Autodesk Inventor part; units mm, degrees
ref_plane "YZ Plane" through (0, 0, 0) normal (1, 0, 0) x (0, 1, 0)
ref_plane "XZ Plane" through (0, 0, 0) normal (0, 1, 0) x (-1, 0, 0)
ref_plane "XY Plane" through (0, 0, 0) normal (0, 0, 1) x (1, 0, 0)
sketch "Skizze1" plane through (0, 0, 0) normal (0, 1, 0) x (-1, 0, 0)
  line L0 (-19.75, -14.75) -> (19.75, -14.75)
  line L1 (19.75, -14.75) -> (19.75, 14.75)
  line L2 (19.75, 14.75) -> (-19.75, 14.75)
  line L3 (-19.75, 14.75) -> (-19.75, -14.75)
  line L4 (0, -20.65) -> (0, 20.65)
  line L5 (27.65, 0) -> (-27.65, 0)
  point P0 (0, 0)
  dimension "d0" = 39.5
  dimension "d1" = 29.5
extrude "Extrusion1" add sketch "Skizze1" along normal blind 6
sketch "Skizze2" plane through (0, 6, 0) normal (0, 1, 0) x (1, 0, 0)
  line L0 (19.75, 14.75) -> (-19.75, 14.75)
  line L1 (-19.75, 14.75) -> (-11.75, 14.75)
  line L2 (-12, 12.75) -> (-12, 7)
  line L3 (-12, 7) -> (-17.75, 7)
  line L4 (-19.75, 6.75) -> (-19.75, 14.75)
  line L5 (19.75, 14.75) -> (10.75, 14.75)
  line L6 (12, 12.75) -> (12, 7)
  line L7 (12, 7) -> (17.75, 7)
  line L8 (19.75, 10.8731) -> (19.75, 14.75)
  line L9 (-19.75, -14.75) -> (19.75, -14.75)
  line L10 (-19.75, -14.75) -> (-11.75, -14.75)
  line L11 (-12, -12.75) -> (-12, -7)
  line L12 (-12, -7) -> (-17.75, -7)
  line L13 (-19.75, -6.75) -> (-19.75, -14.75)
  line L14 (19.75, -14.75) -> (11.75, -14.75)
  line L15 (12, -12.75) -> (12, -7)
  line L16 (12, -7) -> (17.75, -7)
  line L17 (19.75, -6.75) -> (19.75, -14.75)
  circle A0 centre (-14.75, 9.75) radius 1.75
  circle A1 centre (-14.75, -9.75) radius 1.75
  circle A2 centre (14.75, -9.75) radius 1.75
  circle A3 centre (14.75, 9.75) radius 1.75
  line L18 (-19.75, 14.75) -> (-19.75, -14.75)
  line L19 (-19.75, 14.75) -> (19.75, 14.75)
  line L20 (19.75, 14.75) -> (19.75, -14.75)
  line L21 (19.75, -14.75) -> (-19.75, -14.75)
  line L22 (-19.75, -14.75) -> (-19.75, 14.75)
  line L23 (17.75, 12.75) -> (-17.75, 12.75)
  line L24 (-17.75, 12.75) -> (-17.75, -12.75)
  line L25 (-17.75, -12.75) -> (17.75, -12.75)
  line L26 (17.75, 12.75) -> (17.75, -12.75)
  point P0 (0, 0)
  dimension "d12" = 3.5
  dimension "d13" = 5
  dimension "d14" = 5
  dimension "d15" = 3.5
  dimension "d16" = 5
  dimension "d17" = 5
  dimension "d18" = 3.5
  dimension "d19" = 5
  dimension "d20" = 5
  dimension "d21" = 3.5
  dimension "d22" = 5
  dimension "d23" = 5
  dimension "d24" = 2
  dimension "d25" = 2
  dimension "d28" = 2
  dimension "d29" = 2
  dimension "d30" = 7.75
  dimension "d31" = 7.75
  dimension "d35" = 7.75
  dimension "d36" = 7.75
  dimension "d37" = 7.75
  dimension "d38" = 7.75
  dimension "d39" = 7.75
  dimension "d40" = 7.75
sketch "Skizze3" plane through (0, 6, 0) normal (0, 1, 0) x (1, 0, 0)
  circle A0 centre (5.25, 0) radius 7.7
  line L0 (19.75, -14.75) -> (19.75, 14.75)
  line L1 (19.75, 14.75) -> (-19.75, 14.75)
  point P0 (0, 0)
  dimension "d32" = 15.4
  dimension "d33" = 14.5
  dimension "d34" = 14.75
extrude "Extrusion2" add sketch "Skizze2" along normal blind 31.5 contours L8 L20 L17 L9 L13 L18 L4 L0
extrude "Extrusion3" cut sketch "Skizze3" against normal blind 4
sketch "Skizze4" plane through (5.25, 2, 0) normal (0, 1, 0) x (1, 0, 0)
  circle A0 centre (0, 0) radius 5.3
  point P0 (-5.25, 0)
  dimension "d45" = 10.6
extrude "Extrusion4" cut sketch "Skizze4" against normal up to surface (2 mm away)
extrude "Extrusion5" add sketch "Skizze2" along normal blind 31.5 contours L26 L25 L15 L16
extrude "Extrusion6" add sketch "Skizze2" along normal blind 31.5 contours L2 L3 L24 L23 | L23 L26 L7 L6 | L12 L11 L25 L24
extrude "Extrusion7" cut sketch "Skizze2" against normal up to surface (6 mm away) contours A0 | A1 | A2 | A3
fillet "Rundung1" radius 3.5 4 edges at (-12, 21.75, -7) (12, 21.75, -7) (-12, 21.75, 7) (12, 21.75, 7)
fillet "Rundung2" radius 4 4 edges at (19.75, 18.75, 14.75) (19.75, 18.75, -14.75) (-19.75, 18.75, -14.75) (-19.75, 18.75, 14.75)
sketch "Skizze5" plane through (-15.75, 0, 14.75) normal (0, 0, 1) x (1, 0, 0)
  line L0 (3.75, 34) -> (27.75, 34)
  line L1 (27.75, 34) -> (27.75, 17.5)
  line L2 (27.75, 17.5) -> (3.75, 17.5)
  line L3 (3.75, 17.5) -> (3.75, 34)
  line L4 (0, 37.5) -> (31.5, 37.5)
  line L5 (-4, 37.5) -> (-4, 0)
  line L6 (35.5, 0) -> (35.5, 37.5)
  point P0 (15.75, 0)
  dimension "d56" = 16.5
  dimension "d57" = 3.5
  dimension "d58" = 7.75
  dimension "d59" = 7.75
sketch "Skizze6" plane through (15.75, 0, -14.75) normal (0, 0, -1) x (-1, 0, 0)
  line L0 (31.25, 6) -> (27.75, 6)
  line L1 (3.75, 34) -> (27.75, 34)
  line L2 (27.75, 34) -> (27.75, 6)
  line L3 (27.75, 6) -> (3.75, 6)
  line L4 (3.75, 6) -> (3.75, 34)
  line L5 (0, 37.5) -> (31.5, 37.5)
  point P0 (15.75, 0)
  dimension "d60" = 3.5
extrude "Extrusion8" cut sketch "Skizze6" against normal up to surface (2 mm away)
extrude "Extrusion9" cut sketch "Skizze5" against normal up to surface (2 mm away)
sketch "Skizze7" plane through (-19.75, 0, -10.75) normal (-1, 0, 0) x (0, 0, 1)
  line L0 (3.25, 34) -> (17.25, 34)
  line L1 (17.25, 34) -> (17.25, 17.5)
  line L2 (17.25, 17.5) -> (3.25, 17.5)
  line L3 (3.25, 17.5) -> (3.25, 34)
  line L4 (-4, 37.5) -> (-4, 0)
  line L5 (0, 37.5) -> (21.5, 37.5)
  point P0 (10.75, 0)
  dimension "d65" = 14
  dimension "d66" = 16.5
  dimension "d67" = 7.25
  dimension "d68" = 3.5
extrude "Extrusion10" cut sketch "Skizze7" against normal up to surface (2 mm away)
sketch "Skizze8" plane through (19.75, 0, 10.75) normal (1, 0, 0) x (0, 0, -1)
  line L0 (3.25, 34) -> (17.25, 34)
  line L1 (17.25, 34) -> (17.25, 17.5)
  line L2 (17.25, 17.5) -> (3.25, 17.5)
  line L3 (3.25, 17.5) -> (3.25, 34)
  line L4 (-4, 37.5) -> (-4, 0)
  line L5 (0, 37.5) -> (21.5, 37.5)
  point P0 (10.75, 0)
  dimension "d71" = 14
  dimension "d72" = 16.5
  dimension "d73" = 7.25
  dimension "d74" = 3.5
extrude "Extrusion11" cut sketch "Skizze8" against normal up to surface (2 mm away)
sketch "Skizze12" plane through (15.75, 0, -14.75) normal (0, 0, -1) x (-1, 0, 0)
  line L0 (27.75, 34) -> (3.75, 34)
  line L1 (27.75, 6) -> (27.75, 37.5)
  line L2 (3.75, 34) -> (27.75, 34)
  line L3 (27.75, 34) -> (27.75, 37.5)
  line L4 (27.75, 37.5) -> (3.75, 37.5)
  line L5 (3.75, 37.5) -> (3.75, 34)
  point P0 (15.75, 0)
extrude "Extrusion14" cut sketch "Skizze12" against normal up to surface (2 mm away)
sketch "Skizze13" plane through (12, 37.5, 12.75) normal (0, 0, -1) x (-1, 0, 0)
  line L0 (0, 0) -> (0, -31.5)
  line L1 (24, -31.5) -> (24, 0)
  line L2 (0, -3.5027) -> (24, -3.5027)
  line L3 (24, -3.5027) -> (24, 0)
  line L4 (24, 0) -> (0, 0)
  line L5 (0, 0) -> (0, -3.5027)
  point P0 (12, -37.5)
  point P1 (24, -3.5027)
extrude "Extrusion15" cut sketch "Skizze13" against normal up to surface (2 mm away)
sketch "Skizze14" plane through (-15.75, 0, 14.75) normal (0, 0, 1) x (1, 0, 0)
  line L0 (3.75, 6) -> (3.75, 17.5)
  line L1 (27.75, 17.5) -> (27.75, 6)
  line L2 (3.75, 17.5) -> (27.75, 17.5)
  line L3 (27.75, 17.5) -> (27.75, 6)
  line L4 (27.75, 6) -> (3.75, 6)
  line L5 (3.75, 6) -> (3.75, 17.5)
  point P0 (15.75, 0)
  point P1 (27.75, 17.5)
extrude "Extrusion16" cut sketch "Skizze14" against normal up to surface (2 mm away)
sketch "Skizze15" plane through (-19.75, 0, -10.75) normal (-1, 0, 0) x (0, 0, 1)
  point P0 (10.75, 0)
sketch "Skizze16" plane through (-17.75, 6, 7) normal (1, 0, 0) x (0, 0, -1)
  line L0 (14, 0) -> (0, 0)
  line L1 (14, 11.5) -> (14, 28)
  line L2 (0, 0) -> (14, 0)
  line L3 (14, 0) -> (14, 11.5)
  line L4 (14, 11.5) -> (0, 11.5)
  line L5 (0, 11.5) -> (0, 0)
  line L6 (0, 31.5) -> (14, 31.5)
  line L7 (14, 28) -> (0, 28)
  line L8 (0, 28) -> (0, 31.5)
  line L9 (0, 31.5) -> (14, 31.5)
  line L10 (14, 31.5) -> (14, 28)
  point P0 (7, -6)
extrude "Extrusion17" cut sketch "Skizze16" against normal up to surface (2 mm away) contours L7 L8 L6 L10
extrude "Extrusion18" cut sketch "Skizze16" against normal up to surface (2 mm away) contours L0 L5 L4 L3
sketch "Skizze17" plane through (-17.75, 34, 6.5) normal (0, 0, -1) x (-1, 0, 0)
  line L0 (0, 0) -> (2, 0)
  line L1 (2, 0) -> (2, -16.5)
  line L2 (0, 0) -> (2, 0)
  line L3 (2, 0) -> (2, -16.5)
  line L4 (2, -16.5) -> (0, -16.5)
  line L5 (0, -16.5) -> (0, 0)
  point P0 (-17.75, -34)
extrude "Extrusion19" cut sketch "Skizze17" against normal blind 0.5
sketch "Skizze18" plane through (17.75, 6, -7) normal (-1, 0, 0) x (0, 0, 1)
  line L0 (14, 28) -> (14, 31.5)
  line L1 (0.5, 28) -> (14, 28)
  line L2 (14, 31.5) -> (0.5, 31.5)
  line L3 (0.5, 31.5) -> (0.5, 28)
  line L4 (0.5, 28) -> (14, 28)
  line L5 (14, 28) -> (14, 31.5)
  line L6 (14, 0) -> (0, 0)
  line L7 (14.5, 11.5) -> (14, 11.5)
  line L8 (0, 0) -> (14, 0)
  line L9 (14, 0) -> (14, 11.5)
  line L10 (14, 11.5) -> (0, 11.5)
  line L11 (0, 11.5) -> (0, 0)
  point P0 (7, -6)
extrude "Extrusion20" cut sketch "Skizze18" against normal up to surface (2 mm away) contours L6 L11 L10 L9
extrude "Extrusion21" cut sketch "Skizze18" against normal up to surface (2 mm away) contours L1 L3 L2 L0
sketch "Skizze19" plane through (17.75, 37.5, -6.5) normal (0, 0, 1) x (1, 0, 0)
  line L0 (0, -20) -> (0, 0)
  line L1 (2, 0) -> (2, -20)
  line L2 (0, -20) -> (2, -20)
  line L3 (2, -20) -> (2, 0)
  line L4 (2, 0) -> (0, 0)
  line L5 (0, 0) -> (0, -20)
  point P0 (-17.75, -37.5)
extrude "Extrusion22" cut sketch "Skizze19" against normal blind 0.5
properties part number "_3D-Druck"
Verification items for the finished model (mm, model axes). A direction names the side the tool comes from. Give positions to 0.01 mm unless a question says otherwise; leave off trailing zeros. Write each loop counter-clockwise with the first axis right and the second up, starting at its lowest first coordinate (ties: lowest second). Pieces come first, ordered by that corner, then holes. Notation, with made-up numbers: (40.5, -11) - (90.5, -11) arc R14 cw to (90.5, 6) - close; hole circle Ø8 at (-10.75, 89.5). An arc over 180 degrees is marked (long way). Answer as CSV lines item,"result". Start each with the question number.
1. Depth check by flat-ended pin: pin 1 (2 mm diameter, centred on x = -17, y = 20, fed in from -Z); pin 2 (2 mm diameter, centred on x = 17, y = 17.5, fed in from +Z); pin 3 (0.6 mm diameter, centred on x = 18.5, y = 24.5, fed in from -Z). Enter the tip coordinate at first touch or a pass-through.
2. Thickness scan on line 1 (Z direction, x = 5, y = 3); line 2 (Z direction, x = -14, y = 12); line 3 (X direction, y = 10.5, z = 9.75). Record the ranges inside material, lowest first.
3. Sectioned sample at A-A (y = 29.5). Count the separate pieces of the cut face and the enclosed holes in it, then the cut area to 3 significant figures.
4. Sectioned sample at D-D (x = -14.5). Record the boundary of the cut face in (y, z).
5. Draft check along Z on faces 5 (the face through (3.581, 4.028, 7.517)), 6 (the face through (-5, 6, 0)), 7 (the face through (-18.547, 19.012, -13.609)), 8 (the face through (-16, 37.5, 12)). Enter one of: pulls with the +Z half, pulls with the -Z half, needs draft (parallel to the pull), parting line crosses it, or undercut.
6. Sectioned sample at B-B (z = 0). Record the boundary of the cut face in (x, y).
7. Sectioned sample at C-C (x = 5.25). Record the boundary of the cut face in (y, z).
8. Set-up check for faces 1 (the face through (-18, 22, 7)), 2 (the face through (-12, 22, 13)), 3 (the face through (13.05, 21.97, 8)), 4 (the face through (-13.809, 18.488, 11.226)): record each of +Z, -Z, +X, -X, +Y, -Y from which the full face is reachable in a straight line by a thin tool's end or side.
Derived:
1,pin 1,"z = -14.74"
1,pin 2,"z = 14.74"
1,pin 3,"z = -13.91"
2,line 1,"-14.75 to -7.7, 7.7 to 14.75"
2,line 2,"-14.75 to -11.33, -8.17 to -7.34, 7.34 to 8.17, 11.33 to 14.75"
2,line 3,"-19.75 to -16.5, -13 to -12.08, 12.08 to 13, 16.5 to 19.75"
3,separate pieces,"4"
3,enclosed holes,"4"
3,area,"176 mm²"
4,outline,"(0, -14.75) - (37.5, -14.75) - (37.5, -11.48) - (0, -11.48) - close; (0, -8.02) - (37.5, -8.02) - (37.5, -7.15) - (6, -7.15) - (6, 7.15) - (37.5, 7.15) - (37.5, 8.02) - (0, 8.02) - close; (0, 11.48) - (37.5, 11.48) - (37.5, 14.75) - (0, 14.75) - close"
5,face 5,"undercut"
5,face 6,"undercut"
5,face 7,"pulls with the -Z half"
5,face 8,"needs draft"
6,outline,"(-19.75, 0) - (-0.05, 0) - (-0.05, 2) - (-2.45, 2) - (-2.45, 6) - (-19.75, 6) - close; (10.55, 0) - (19.75, 0) - (19.75, 6) - (12.95, 6) - (12.95, 2) - (10.55, 2) - close"
7,outline,"(0, -14.75) - (6, -14.75) - (6, -7.7) - (2, -7.7) - (2, -5.3) - (0, -5.3) - close; (0, 5.3) - (2, 5.3) - (2, 7.7) - (6, 7.7) - (6, 14.75) - (0, 14.75) - close"
8,face 1,"+X, -X, +Y"
8,face 2,"+Z, -Z, +Y"
8,face 3,"+Y"
8,face 4,"+Y, -Y"
